```python
from build123d import *

# Parameters (mm, degrees)
SKETCH1_R           = 7.5
BOSS_EXTRUDE1_DEPTH = 25
SKETCH2_R           = 10
BOSS_EXTRUDE2_DEPTH = 2.5
BOSS_EXTRUDE3_START = -7.5
SKETCH2_2_R         = 10
BOSS_EXTRUDE3_DEPTH = 2.5
BOSS_EXTRUDE4_DEPTH = 5
SKETCH5_R           = 10
BOSS_EXTRUDE5_DEPTH = 57.5


with BuildPart() as part:
    # Sketch1 → Boss-Extrude1 (new body)
    with BuildSketch(Plane.XY):
        Circle(SKETCH1_R)
    extrude(amount=BOSS_EXTRUDE1_DEPTH)

    # Sketch2 → Boss-Extrude2 (add)
    with BuildSketch(Plane.XY.offset(25)):
        Circle(SKETCH2_R)
    extrude(amount=-BOSS_EXTRUDE2_DEPTH)

    # Sketch2_2 → Boss-Extrude3 (add)
    with BuildSketch(Plane.XY.offset(25).offset(BOSS_EXTRUDE3_START)):
        Circle(SKETCH2_2_R)
    extrude(amount=-BOSS_EXTRUDE3_DEPTH)

    # Sketch4 → Boss-Extrude4 (add)
    with BuildSketch(Plane(origin=(0, 0, 0), x_dir=(-1, 0, 0), z_dir=(0, 0, -1))):
        with BuildLine():
            Line((-10, 0), (-10, -25))
            ThreePointArc((-10, -25), (0, -35), (10, -25))
            Line((10, -25), (10, 0))
            ThreePointArc((10, 0), (0, 10), (-10, 0))
        make_face()
    extrude(amount=-BOSS_EXTRUDE4_DEPTH)

    # Sketch5 → Boss-Extrude5 (add)
    with BuildSketch(Plane.XY.offset(5)):
        with Locations((0, -25)):
            Circle(SKETCH5_R)
    extrude(amount=-BOSS_EXTRUDE5_DEPTH)

    # Sketch6 → Revolve1 (revolve)
    with BuildSketch(Plane(origin=(0, 0, 0), x_dir=(0, 0, -1), z_dir=(1, 0, 0))):
        with BuildLine():
            Line((52.5, -25), (77.5, -25))
            Line((77.5, -25), (77.5, -15))
            ThreePointArc((77.5, -15), (71.108894336, -6.814422655), (61.617647059, -11.029411765))
            ThreePointArc((61.617647059, -11.029411765), (58.858718166, -13.931196943), (55, -15))
            Line((55, -15), (52.5, -15))
            Line((52.5, -15), (52.5, -25))
        make_face()
    revolve(axis=Axis((0, -25, -52.5), (0, 0, -1)))


solid = part.part
```
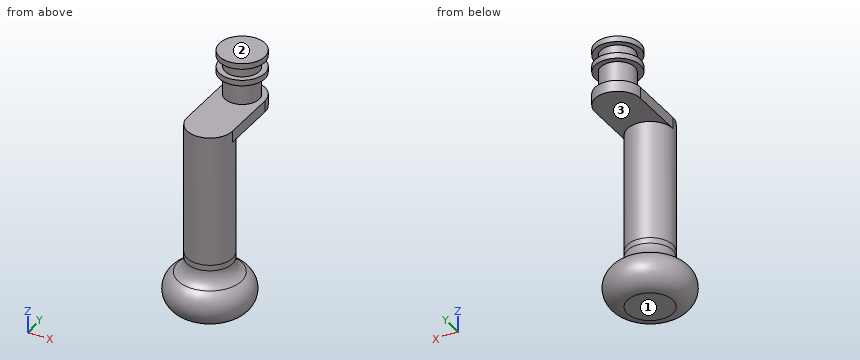
Check sheet for the modelled part. Datum: model origin and axes. Units: mm. Face numbers are marked on the shaded views. Give positions to 0.01 mm unless a question says otherwise; leave off trailing zeros. Order: outer loops, then holes, each group sorted by start corner. A loop starts at its lowest first (then second) coordinate and runs counter-clockwise, first axis right, second up. Notation, with made-up numbers: M 14.5,69.25 L 36.5,69.25 A17 ccw 36.5,82.25 Z; hole C 61.5,10.5 d6. An arc over 180 degrees is marked long. Answer in a Markdown table with one row per item. Add a question column.
Q1. Release check for a two-part mould opening along Z. For the marked faces 1, 2 and 3 record: released by +Z, released by -Z, zero draft, split by the parting line, or undercut.
Q2. Gauge pin test, flat ends, axial feed: pin 1 Ø2.5 at (y, z) = (-10, 3) entering from +X; pin 2 Ø3 at (y, z) = (-22, -29) entering from -X; pin 3 Ø22 at (x, y) = (-3.5, -21.5) entering from +Z; pin 4 Ø3 at (y, z) = (-21.5, 8) entering from -X. Record the tip position at first contact, or that the pin passes through.
Q3. Thickness scan on L1, parallel to Z at x = 6, y = -19.5; L2, parallel to Z at x = -8, y = -16.5; L3, parallel to Z at x = 0.5, y = -1.5. Record the ranges inside material, lowest first.
Q4. Sectioned sample at C-C, the plane y = 3. Record the boundary of the cut face in (x, z), and give its area (3 significant figures).
Q5. Sectioned sample at B-B, the plane z = -38. Record the boundary of the cut face in (x, y).
Q6. Sectioned sample at D-D, the plane y = -5. Record the boundary of the cut face in (x, z), and give its area (3 significant figures).
Q7. Sectioned sample at A-A, the plane x = 0. Record the boundary of the cut face in (y, z) (1 decimal).
Verdict:
| question | item | result |
|---|---|---|
| 1 | face 1 | released by -Z |
| 1 | face 2 | released by +Z |
| 1 | face 3 | undercut |
| 2 | pin 1 | x = 10 |
| 2 | pin 2 | x = -9.89 |
| 2 | pin 3 | z = 5 |
| 2 | pin 4 | through |
| 3 | L1 | -77.5 to 5 |
| 3 | L2 | -77.33 to -59.72, 0 to 5 |
| 3 | L3 | 0 to 25 |
| 4 | outline | M -9.54,0 L 9.54,0 L 9.54,5 L 6.87,5 L 6.87,15 L 9.54,15 L 9.54,17.5 L 6.87,17.5 L 6.87,22.5 L 9.54,22.5 L 9.54,25 L -9.54,25 L -9.54,22.5 L -6.87,22.5 L -6.87,17.5 L -9.54,17.5 L -9.54,15 L -6.87,15 L -6.87,5 L -9.54,5 Z |
| 4 | area | 397 mm² |
| 5 | outline | C 0,-25 d20 |
| 6 | outline | M -10,0 L 10,0 L 10,5 L 5.59,5 L 5.59,15 L 8.66,15 L 8.66,17.5 L 5.59,17.5 L 5.59,22.5 L 8.66,22.5 L 8.66,25 L -8.66,25 L -8.66,22.5 L -5.59,22.5 L -5.59,17.5 L -8.66,17.5 L -8.66,15 L -5.59,15 L -5.59,5 L -10,5 Z |
| 6 | area | 354 mm² |
| 7 | outline | M -39,-61.6 A8.4 ccw -35,-77.5 L -15,-77.5 A8.4 ccw -11,-61.6 A7.5 cw -15,-55 L -15,0 L 10,0 L 10,5 L 7.5,5 L 7.5,15 L 10,15 L 10,17.5 L 7.5,17.5 L 7.5,22.5 L 10,22.5 L 10,25 L -10,25 L -10,22.5 L -7.5,22.5 L -7.5,17.5 L -10,17.5 L -10,15 L -7.5,15 L -7.5,5 L -35,5 L -35,-55 A7.5 cw Z |
